Design review of the part built by this model. Coordinates are the model's own, in mm. Face numbers are marked on the shaded views. A direction names the side the tool comes from. Coordinates: 2 decimals unless noted, no trailing zeros. Loops run counter-clockwise (first coordinate to the right, second up) from the corner with the lowest first, then second, coordinate; pieces in that order, holes last. Notation, with made-up numbers: M 50,53.25 L 63,53.25 A29 cw 63,81.25 Z; hole C 29,76 d4. An arc over 180 degrees is marked long. Put each result on its own line as item: value. Start each with the question number.
(1) Take a section at A-A, the plane y = -11. Give the boundary of the cut face in (x, z).
(2) For the marked faces 1, 2, 3, 4 and 5, list the 3-axis set-ups (+Z, -Z, +X, -X, +Y, -Y) from which the entire face can be reached by the end or side of a thin tool; tool diameter is ignored.
(3) Clearance check with flat-ended pins moving along their axes: pin 1 (1 mm diameter, centred on x = -45.5, z = 33.5, fed in from +Y); pin 2 (1 mm diameter, centred on x = 9, y = -63.5, fed in from -Z); pin 3 (13.5 mm diameter, centred on y = -125.5, z = 11, fed in from -X). State where each tip first meets the part, or that it passes through.
(4) For probe 1 along X at (y, z) = (-118.5, 14.5); probe 2 along X at (y, z) = (-23.5, -17); probe 3 along Z at (x, y) = (33, -28), list the stretches that pass through material, from the lowest coordinate up. Write a range as [from, to].
(5) Take a section at B-B, the plane y = -128.5. Give the boundary of the cut face in (x, z), then the cut area to 3 significant figures.
```python
from build123d import *

# Parameters (mm, degrees)
CROQUIS1_W              = 220
CROQUIS1_H              = 220
SALIENTE_EXTRUIR1_DEPTH = 100
CROQUIS2_OUTSIDE_W      = 437.492
CROQUIS2_OUTSIDE_H      = 437.492
CROQUIS2_OUTSIDE_W_2    = 70
CROQUIS2_OUTSIDE_H_2    = 70
CORTAR_EXTRUIR1_DEPTH   = 70
CORTAR_EXTRUIR1_TAPER   = 47
CROQUIS3_W              = 70
CROQUIS3_H              = 70
SALIENTE_EXTRUIR2_DEPTH = 40
VACIADO1_T              = -10
CROQUIS3_3_W            = 50
CROQUIS3_3_H            = 50
CORTAR_EXTRUIR2_DEPTH   = 40


with BuildPart() as part:
    # Croquis1 → Saliente-Extruir1 (new body)
    with BuildSketch(Plane(origin=(0, 0, 0), x_dir=(1, 0, 0), z_dir=(0, 1, 0))):
        Rectangle(CROQUIS1_W, CROQUIS1_H)
    extrude(amount=-SALIENTE_EXTRUIR1_DEPTH)

    # Croquis2 outside → Cortar-Extruir1 (cut)
    with BuildSketch(Plane.XZ.offset(100)):
        Rectangle(CROQUIS2_OUTSIDE_W, CROQUIS2_OUTSIDE_H)
        Rectangle(CROQUIS2_OUTSIDE_W_2, CROQUIS2_OUTSIDE_H_2, mode=Mode.SUBTRACT)
    extrude(amount=-CORTAR_EXTRUIR1_DEPTH, taper=CORTAR_EXTRUIR1_TAPER, mode=Mode.SUBTRACT)

    # Croquis3 → Saliente-Extruir2 (add)
    with BuildSketch(Plane.XZ.offset(100)):
        Rectangle(CROQUIS3_W, CROQUIS3_H)
    extrude(amount=SALIENTE_EXTRUIR2_DEPTH)

    # Vaciado1
    vaciado1_openings = [part.faces().sort_by_distance(p)[0] for p in [
        (0, 0, 0),
    ]]
    offset(amount=VACIADO1_T, openings=vaciado1_openings, kind=Kind.INTERSECTION)

    # Croquis3<3> → Cortar-Extruir2 (cut)
    with BuildSketch(Plane.XZ.offset(100)):
        Rectangle(CROQUIS3_3_W, CROQUIS3_3_H)
    extrude(amount=CORTAR_EXTRUIR2_DEPTH, mode=Mode.SUBTRACT)


solid = part.part
```
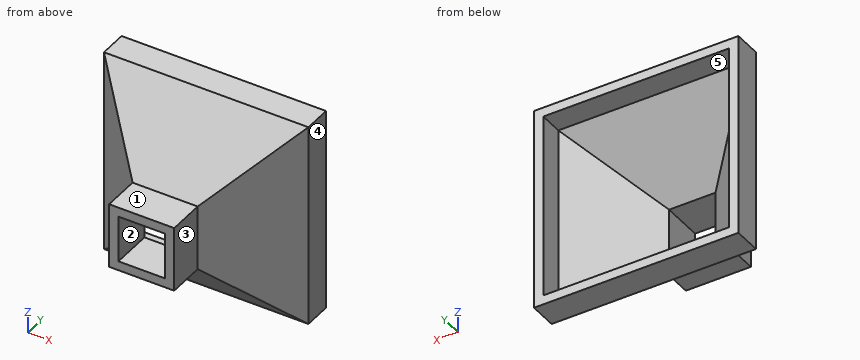
Computed values:
1. outline: M -110,-110 L 110,-110 L 110,110 L -110,110 Z; hole M -100,-100 L 100,-100 L 100,100 L -100,100 Z
2. face 1: +Z, +X, -X, -Y
2. face 2: +Y, -Y
2. face 3: +Z, -Z, +X, -Y
2. face 4: +Z, -Z, +X, +Y, -Y
2. face 5: +Y
3. pin 1: stops at y = -76.07
3. pin 2: stops at z = -74.68
3. pin 3: stops at x = -35
4. probe 1: x = [-35, -25], [25, 35]
4. probe 2: x = [-110, -100], [100, 110]
4. probe 3: z = [-110, -97.55], [97.55, 110]
5. outline: M -35,-35 L 35,-35 L 35,35 L -35,35 Z; hole M -25,-25 L 25,-25 L 25,25 L -25,25 Z
5. area: 2,400 mm^2
